from build123d import *

# Parameters (mm, degrees)
SKETCH1_W           = 215.5
SKETCH1_H           = 201
BOSS_EXTRUDE1_DEPTH = 49
BOSS_EXTRUDE1_DRAFT = -1
FILLET1_R           = 3
CUT_EXTRUDE1_DEPTH  = 45
CUT_EXTRUDE1_DRAFT  = -1


with BuildPart() as part:
    # Sketch1 → Boss-Extrude1 (with draft: the straight prism first)
    with BuildSketch(Plane(origin=(0, 0, 0), x_dir=(1, 0, 0), z_dir=(0, 1, 0))):
        Rectangle(SKETCH1_W, SKETCH1_H)
    extrude(amount=BOSS_EXTRUDE1_DEPTH)
    # Boss-Extrude1: the draft: its side faces are tilted about the plane it starts from
    boss_extrude1_sides = [part.faces().sort_by_distance(p)[0] for p in [
        (0, 24.5, 100.5),
        (107.75, 24.5, 0),
        (0, 24.5, -100.5),
        (-107.75, 24.5, 0),
    ]]
    draft(boss_extrude1_sides, Plane(origin=(0, 0, 0), x_dir=(1, 0, 0), z_dir=(0, 1, 0)), BOSS_EXTRUDE1_DRAFT)

    # Fillet1
    fillet1_edges = [part.edges().sort_by_distance(p)[0] for p in [
        (0, 0, 100.5),
        (-107.75, 0, 0),
        (0, 0, -100.5),
        (107.75, 0, 0),
        (108.177649091, 24.5, 100.927649091),
        (-108.177649091, 24.5, 100.927649091),
        (-108.177649091, 24.5, -100.927649091),
        (108.177649091, 24.5, -100.927649091),
    ]]
    fillet(fillet1_edges, radius=FILLET1_R)


with BuildPart() as cut_extrude1_tool:
    # Sketch2 → Cut-Extrude1 (with draft: the straight prism first)
    with BuildSketch(Plane(origin=(0, 49, 0), x_dir=(1, 0, 0), z_dir=(0, 1, 0))):
        with BuildLine():
            Line((-104.605298181, -99.355298181), (104.605298181, -99.355298181))
            ThreePointArc((104.605298181, -99.355298181), (106.019511744, -98.769511744), (106.605298181, -97.355298181))
            Line((106.605298181, -97.355298181), (106.605298181, 97.355298181))
            ThreePointArc((106.605298181, 97.355298181), (106.019511744, 98.769511744), (104.605298181, 99.355298181))
            Line((104.605298181, 99.355298181), (-104.605298181, 99.355298181))
            ThreePointArc((-104.605298181, 99.355298181), (-106.019511744, 98.769511744), (-106.605298181, 97.355298181))
            Line((-106.605298181, 97.355298181), (-106.605298181, -97.355298181))
            ThreePointArc((-106.605298181, -97.355298181), (-106.019511744, -98.769511744), (-104.605298181, -99.355298181))
        make_face()
    extrude(amount=-CUT_EXTRUDE1_DEPTH)
    # Cut-Extrude1: the draft: its side faces are tilted about the plane it starts from
    cut_extrude1_sides = [cut_extrude1_tool.faces().sort_by_distance(p)[0] for p in [
        (0, 26.5, 99.355298181),
        (106.019511744, 26.5, 98.769511744),
        (106.605298181, 26.5, 0),
        (106.019511744, 26.5, -98.769511744),
        (0, 26.5, -99.355298181),
        (-106.019511744, 26.5, -98.769511744),
        (-106.605298181, 26.5, 0),
        (-106.019511744, 26.5, 98.769511744),
    ]]
    draft(cut_extrude1_sides, Plane(origin=(0, 49, 0), x_dir=(1, 0, 0), z_dir=(0, 1, 0)), CUT_EXTRUDE1_DRAFT)


with BuildPart() as part_1:
    add(part.part)

    # Cut-Extrude1: cut by cut_extrude1_tool
    add(cut_extrude1_tool.part, mode=Mode.SUBTRACT)


solid = part_1.part
Design review of the part built by this model. Coordinates are the model's own, in mm. Give positions to 0.01 mm unless a question says otherwise; leave off trailing zeros. Loops run counter-clockwise (first coordinate to the right, second up) from the corner with the lowest first, then second, coordinate; pieces in that order, holes last. Notation, with made-up numbers: (-19.75, -23) -> (-3.75, -23) arc R25 ccw to (-3.75, -1) -> close; hole circle Ø9 at (76, -1). An arc over 180 degrees is marked (long way). One line per question, with ' | ' between items. Start each with the question number.
(1) Draft analysis for pull direction X (two halves, no side actions). For faces 1 (the face through (-1, 4, -1)), 2 (the face through (-1, 0, -1)), state which applies: +X half, -X half, draft (parallel to the pull), parting line (faces both ways), or undercut.
(2) For line 1 (X direction, y = 47.5, z = 93); line 2 (Z direction, x = 44, y = 45.5); line 3 (Y direction, x = -16, z = -18), list the stretches that pass through material, from the lowest coordinate up.
(3) We need section B-B (x = -69). State the section outline as (y, z) points, and give its area (3 significant figures).
(4) We need section A-A (z = -52.5). State the section outline as (x, y) points.
(5) Insertion check: P1, Ø3, axis at y = 28, z = 63.5, coming from the +X side; P2, Ø10, axis at y = 14, z = -17, coming from the -X side; P3, Ø1, axis at x = -37.5, y = 37.5, coming from the -Z side. Each pin has a flat end and moves straight along its axis. Give the tip position at first contact, or say it passes through.
The answers:
1) face 1: undercut | face 2: draft
2) line 1: x = -108.58 to -106.58, 106.58 to 108.58 | line 2: z = -101.29 to -99.29, 99.29 to 101.29 | line 3: y = 0 to 4
3) outline: (0, -97.55) arc R3 ccw to (2.95, -100.55) -> (49, -101.36) -> (49, -99.36) -> (4, -98.57) -> (4, 98.57) -> (49, 99.36) -> (49, 101.36) -> (2.95, 100.55) arc R3 ccw to (0, 97.55) -> close | area: 981 mm^2
4) outline: (-108.61, 49) -> (-107.8, 2.95) arc R3 ccw to (-104.8, 0) -> (104.8, 0) arc R3 ccw to (107.8, 2.95) -> (108.61, 49) -> (106.61, 49) -> (105.82, 4) -> (-105.82, 4) -> (-106.61, 49) -> close
5) P1: stops at x = 108.26 | P2: stops at x = -108.08 | P3: stops at z = -101.16
